For this review, take the finished solid that the model builds, in its own axes (mm). A direction names the side the tool comes from. Give positions to 0.01 mm unless a question says otherwise; leave off trailing zeros. Order: outer loops, then holes, each group sorted by start corner. A loop starts at its lowest first (then second) coordinate and runs counter-clockwise, first axis right, second up. Notation, with made-up numbers: (80, 88) - (102, 88) arc R18 cw to (102, 119) - close; hole circle Ø1 at (-7.75, 57.5). An arc over 180 degrees is marked (long way). One line per item, written item: value.
Autodesk Inventor part; units mm, degrees
ref_plane "Work Plane1" through (-52.5, 0, -5) normal (1, 0, 0) x (0, 0, -1)
ref_plane "YZ Plane" through (0, 0, 0) normal (1, 0, 0) x (0, 1, 0)
ref_plane "XZ Plane" through (0, 0, 0) normal (0, 1, 0) x (-1, 0, 0)
sketch "Sketch1" plane through (0, 0, 0) normal (0, 1, 0) x (-1, 0, 0)
  line L0 (0, 0) -> (105, 0)
  line L1 (105, 0) -> (105, -105)
  line L2 (105, -105) -> (0, -105)
  line L3 (0, -105) -> (0, 0)
  dimension "d0" = 105
  dimension "d1" = 105
extrude "Extrusion1" add sketch "Sketch1" along normal blind 5
fillet "Fillet1" radius 5 4 edges at (-105, 2.5, -105) (0, 2.5, 0) (0, 2.5, -105) (-105, 2.5, 0)
sketch "Sketch3" plane through (0, 5, 0) normal (0, 1, 0) x (1, 0, 0)
  line L0 (-102.5, 102.5) -> (-2.5, 102.5) construction
  line L1 (-2.5, 102.5) -> (-2.5, 2.5) construction
  line L2 (-2.5, 2.5) -> (-102.5, 2.5) construction
  line L3 (-102.5, 2.5) -> (-102.5, 102.5) construction
  line L4 (0, 5) -> (0, 100)
  line L5 (-5, 105) -> (-100, 105)
  line L6 (-105, 100) -> (-105, 5)
  line L7 (-100, 0) -> (-5, 0)
  point P0 (0, 0)
  dimension "d11" = 2.5
  dimension "d12" = 2.5
  dimension "d13" = 2.5
  dimension "d14" = 2.5
sketch "Sketch4" plane through (0, 5, 0) normal (0, 1, 0) x (1, 0, 0)
  line L0 (-101, 101) -> (-4, 101) construction
  line L1 (-4, 101) -> (-4, 4) construction
  line L2 (-4, 4) -> (-101, 4) construction
  line L3 (-101, 4) -> (-101, 101) construction
  line L4 (0, 5) -> (0, 100)
  line L5 (-105, 100) -> (-105, 5)
  line L6 (-100, 0) -> (-5, 0)
  line L7 (-5, 105) -> (-100, 105)
  circle A0 centre (-101, 101) radius 1.5
  circle A1 centre (-4, 101) radius 1.5
  circle A2 centre (-4, 4) radius 1.5
  circle A3 centre (-101, 4) radius 1.5
  point P0 (0, 0)
  dimension "d15" = 4
  dimension "d16" = 4
  dimension "d17" = 4
  dimension "d18" = 4
  dimension "d19" = 3
  dimension "d20" = 3
  dimension "d21" = 3
  dimension "d22" = 3
extrude "Extrusion3" cut sketch "Sketch4" against normal blind 10
sketch "Sketch5" plane through (0, 5, 0) normal (0, 1, 0) x (1, 0, 0)
  circle A0 centre (-4, 4) radius 1.5
  line L0 (-5.5, 4) -> (-5.5, 101)
  circle A1 centre (-4, 101) radius 1.5
  line L1 (-2.5, 101) -> (-2.5, 4)
  circle A2 centre (-101, 4) radius 1.5
  circle A3 centre (-101, 101) radius 1.5
  point P0 (0, 0)
extrude "Extrusion4" cut sketch "Sketch5" against normal blind 10 contours A0 | A0 L0 A1 L1 | A1
ref_plane "Work Plane1" through (-52.5, 0, -5) normal (1, 0, 0) x (0, 0, -1)
mirror "Mirror1" about plane through (-52.5, 0, -5) normal (1, 0, 0) of "Extrusion4"
properties part number "Adult fly trap top and bottom"
(1) Machinability: for faces 1 (the face through (-1, 3, -103)), 2 (the face through (-99.5, 3, -53)), which of the approach directions +Z, -Z, +X, -X, +Y, -Y give a long, thin tool a straight path to every point of the face, cutting with its end or side? Answer none if there is none.
Answers below:
face 1: -Z, +X, +Y, -Y
face 2: +Y, -Y
(2) Take a section at A-A (y = 2.4). Write out the cut boundary in (x, z).
Answers below:
outline: (-105, -100) arc R5 ccw to (-100, -105) - (-5, -105) arc R5 ccw to (0, -100) - (0, -5) arc R5 ccw to (-5, 0) - (-100, 0) arc R5 ccw to (-105, -5) - close; hole (-102.5, -101) arc R1.5 ccw to (-99.5, -101) - (-99.5, -4) arc R1.5 ccw to (-102.5, -4) - close; hole (-5.5, -101) arc R1.5 ccw to (-2.5, -101) - (-2.5, -4) arc R1.5 ccw to (-5.5, -4) - close
(3) Take a section at B-B (z = -47). Write out the cut boundary in (x, y), then the cut area to 3 significant figures.
Answers below:
outline: (-105, 0) - (-102.5, 0) - (-102.5, 5) - (-105, 5) - close; (-99.5, 0) - (-5.5, 0) - (-5.5, 5) - (-99.5, 5) - close; (-2.5, 0) - (0, 0) - (0, 5) - (-2.5, 5) - close
area: 495 mm^2
(4) For P1, Ø2, axis at x = -63, y = 4.5, coming from the +Z side, flat-tipped, find the tip position at first contact; note if it passes through.
Answers below:
P1: stops at z = 0
(5) Draft analysis for pull direction X (two halves, no side actions). For faces 3 (the face through (-102.5, 3, -52)), 4 (the face through (0, 2, -53)), 5 (the face through (-53, 2, -105)), 6 (the face through (-4, 2.5, -102.5)), state which applies: pulls with the +X half, pulls with the -X half, needs draft (parallel to the pull), parting line crosses it, or undercut.
Answers below:
face 3: undercut
face 4: pulls with the +X half
face 5: needs draft
face 6: undercut
(6) Wall thickness on line 1 (X direction, y = 3.5, z = -98.5): over which ranges is the line inside the solid? List them lowest first. Write a range as from..to.
Answers below:
line 1: x = -105..-102.5, -99.5..-5.5, -2.5..0
